Geometry check sheet. Reference: the model listing, model coordinates, mm. A direction names the side the tool comes from. Coordinates: 2 decimals unless noted, no trailing zeros. Order: outer loops, then holes, each group sorted by start corner. A loop starts at its lowest first (then second) coordinate and runs counter-clockwise, first axis right, second up. Notation, with made-up numbers: (42, -22.5) - (81, -22.5) arc R22 ccw to (81, 9.5) - close; hole circle Ø3 at (51.25, 61). An arc over 180 degrees is marked (long way). Return JSON: item names as keys, results as strings. Group by question number.
Item 1: Section check C-C on x = 33. Enter the section's corners in (y, z) (3 decimals).
Item 2: Gauge pin test, flat ends, axial feed: pin 1 (10.5 mm diameter, centred on x = 17.96, z = -17.96, fed in from -Y) (3 decimals); pin 2 (10 mm diameter, centred on y = 1, z = -9, fed in from -X); pin 3 (4 mm diameter, centred on x = 4.5, y = 3.5, fed in from -Z); pin 4 (3 mm diameter, centred on y = 0.5, z = -16.5, fed in from -X). Record the tip position at first contact, or that the pin passes through.
Item 3: Section check D-D on y = 3. Enter the section's corners in (x, z) (1 decimal), then the cut area to 3 significant figures.
Item 4: Tool access check on faces 1 (the flat face through (22.806, 6.277, -8.745)), 2 (the flat face through (17, 9.525, -22)). Record the directions out of +Z, -Z, +X, -X, +Y, -Y that give a thin tool (end or side, any length) a straight path to the whole face; none if there is none.
Item 5: Section check A-A on y = 7.5. Enter the section's corners in (x, z) (1 decimal).
Item 6: Section check B-B on z = -20.5. Give the number of separate pieces and of enclosed holes in the cut face, then the cut area to 3 significant figures.
Item 7: Draft check along Z on faces 3 (the flat face through (8.71, 6.28, -22.84)), 4 (the flat face through (17, -9.525, -22)), 5 (the cylindrical face through (0.708, -0.133, -31.205)). Enter one of: pulls with the +Z half, pulls with the -Z half, needs draft (parallel to the pull), parting line crosses it, or undercut.
Item 8: Scan lines: probe 1 along X at (y, z) = (-1, -16); probe 2 along Z at (x, y) = (19.5, 0); probe 3 along X at (y, z) = (4.5, -18). Record each from-to range of solid material in increasing order.
from build123d import *

# Parameters (mm, degrees)
SKETCH2_R           = 3.302
BOSS_EXTRUDE2_DEPTH = 9.525
SKETCH4_R           = 1.950000037
CUT_EXTRUDE2_DEPTH  = 5.800000084
FILLET1_R           = 8.255


with BuildPart() as part:
    # Sketch2 → Boss-Extrude2 (new body, symmetric)
    with BuildSketch(Plane(origin=(0, 0, 0), x_dir=(1, 0, 0), z_dir=(0, 1, 0))):
        with BuildLine():
            Line((-11.353721197, 34.702387112), (34.702387112, -11.353721197))
            ThreePointArc((34.702387112, -11.353721197), (25.818236348, 25.818236348), (-11.353721197, 34.702387112))
        make_face()
        with Locations((17.960512242, 17.960512242)):
            Circle(SKETCH2_R, mode=Mode.SUBTRACT)
    extrude(amount=BOSS_EXTRUDE2_DEPTH, both=True)

    # Sketch4 → Cut-Extrude2 (cut)
    with BuildSketch(Plane(origin=(11.674332957, 0, -11.674332957), x_dir=(0.707106781, 0, 0.707106781), z_dir=(-0.707106781, 0, 0.707106781))):
        with Locations((9.969999999, 6.249999946)):
            Circle(SKETCH4_R)
        with Locations((-9.969999999, 6.249999946)):
            Circle(SKETCH4_R)
        with Locations((-9.969999999, -6.249999946)):
            Circle(SKETCH4_R)
        with Locations((9.969999999, -6.249999946)):
            Circle(SKETCH4_R)
    extrude(amount=-CUT_EXTRUDE2_DEPTH, mode=Mode.SUBTRACT)

    # Fillet1
    fillet1_edges = [part.edges().sort_by_distance(p)[0] for p in [
        (34.702387112, 0, 11.353721197),
        (-11.353721197, 0, -34.702387112),
    ]]
    fillet(fillet1_edges, radius=FILLET1_R)


solid = part.part
Computed:
{
 "1": {"outline": "(-9.525, -15.626) - (9.525, -15.626) - (9.525, -2.081) - (-9.525, -2.081) - close"},
 "2": {"pin 1": "stops at y = -9.525", "pin 2": "stops at x = 9.35", "pin 3": "stops at z = -35.27", "pin 4": "stops at x = 5.35"},
 "3": {"outline": "(2.1, -21.3) arc R8.3 ccw to (10.2, -35.1) arc R36.5 ccw to (35.1, -10.2) arc R8.3 ccw to (21.3, -2.1) - close; hole circle Ø6.6 at (18, -18)", "area": "703 mm²"},
 "4": {"face 1": "none", "face 2": "+Z, -Z, +X, -X, +Y"},
 "5": {"outline": "(2.1, -21.3) arc R8.3 ccw to (10.2, -35.1) arc R36.5 ccw to (35.1, -10.2) arc R8.3 ccw to (21.3, -2.1) - (19.8, -3.6) - (23.9, -7.7) - (21.8, -9.8) - (17.7, -5.7) - (5.7, -17.7) - (9.8, -21.8) - (7.7, -23.9) - (3.6, -19.8) - close; hole circle Ø6.6 at (18, -18)"},
 "6": {"separate pieces": "2", "enclosed holes": "2", "area": "407 mm²"},
 "7": {"face 3": "undercut", "face 4": "needs draft", "face 5": "parting line crosses it"},
 "8": {"probe 1": "x = 7.35 to 15.3, 20.62 to 32.82", "probe 2": "z = -30.87 to -20.88, -15.04 to -3.85", "probe 3": "x = 5.35 to 14.66, 21.26 to 31.77"}
}
